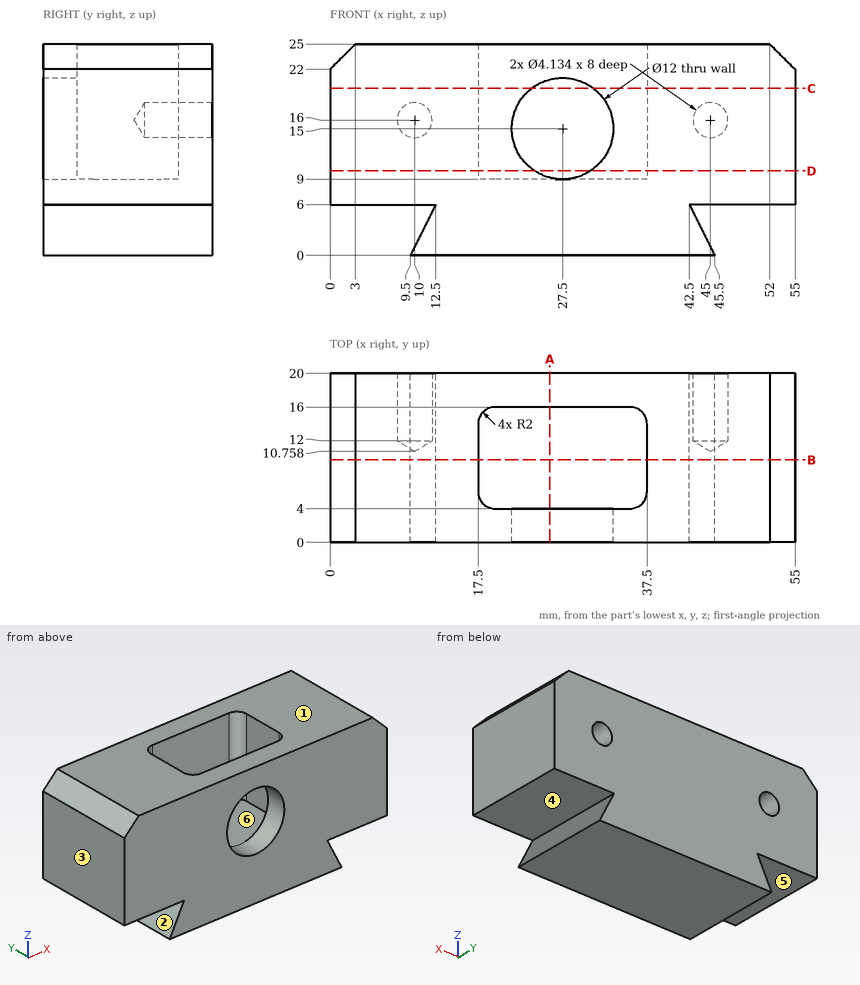
Geometry: see drawing. Coordinates: mm, zero at the bounding-box minimum. A direction names the side the tool comes from. Give positions to 0.01 mm unless a question says otherwise; leave off trailing zeros. Order: outer loops, then holes, each group sorted by start corner. A loop starts at its lowest first (then second) coordinate and runs counter-clockwise, first axis right, second up. Notation, with made-up numbers: (-2, -39) -> (13, -39) arc R14 ccw to (13, -16) -> close; hole circle Ø8 at (-4.5, 28.25). An arc over 180 degrees is marked (long way). Write item = value, one per line.
Q1. Cut plane A-A, the plane x = 26. Output: boundary loops of the cut face in (y, z).
Data:
outline = (0, 0) -> (20, 0) -> (20, 25) -> (16, 25) -> (16, 9) -> (4, 9) -> (4, 9.19) -> (0, 9.19) -> close; (0, 20.81) -> (4, 20.81) -> (4, 25) -> (0, 25) -> close
Q2. Material intervals for line 1 (X direction, y = 14, z = 16); line 2 (X direction, y = 16.25, z = 16); line 3 (Y direction, x = 23, z = 24), sorted ascending. Write a range as from..to.
Data:
line_1 = 0..7.93, 12.07..17.5, 37.5..42.93, 47.07..55
line_2 = 0..7.93, 12.07..42.93, 47.07..55
line_3 = 0..4, 16..20
Q3. Pull-direction query (Z, two-part tool) for the marked faces 1, 2 and 3; classes: released by +Z, released by -Z, zero draft, split by the parting line, or undercut.
Data:
face_1 = released by +Z
face_2 = undercut
face_3 = zero draft
Q4. Pin query (flat end, axial travel): pin 1 (9.5 mm diameter, centred on x = 26, y = 10.5, fed in from +Z); pin 2 (1 mm diameter, centred on y = 7, z = 4.5, fed in from -X). Return the tip coordinate at first contact, or that it passes through.
Data:
pin_1 = 9
pin_2 = 11.5
Q5. Cut plane D-D, the plane z = 10. Output: boundary loops of the cut face in (x, y).
Data:
outline = (0, 0) -> (24.18, 0) -> (24.18, 4) -> (19.5, 4) arc R2 cw to (17.5, 6) -> (17.5, 14) arc R2 cw to (19.5, 16) -> (35.5, 16) arc R2 cw to (37.5, 14) -> (37.5, 6) arc R2 cw to (35.5, 4) -> (30.82, 4) -> (30.82, 0) -> (55, 0) -> (55, 20) -> (0, 20) -> close
Q6. Cut plane B-B, the plane y = 9.75. Output: boundary loops of the cut face in (x, z).
Data:
outline = (0, 6) -> (12.5, 6) -> (9.5, 0) -> (45.5, 0) -> (42.5, 6) -> (55, 6) -> (55, 22) -> (52, 25) -> (37.5, 25) -> (37.5, 9) -> (17.5, 9) -> (17.5, 25) -> (3, 25) -> (0, 22) -> close
Q7. Cut plane C-C, the plane z = 19.75. Output: boundary loops of the cut face in (x, y).
Data:
outline = (0, 0) -> (23.83, 0) -> (23.83, 4) -> (19.5, 4) arc R2 cw to (17.5, 6) -> (17.5, 14) arc R2 cw to (19.5, 16) -> (35.5, 16) arc R2 cw to (37.5, 14) -> (37.5, 6) arc R2 cw to (35.5, 4) -> (31.17, 4) -> (31.17, 0) -> (55, 0) -> (55, 20) -> (0, 20) -> close
Q8. Set-up query: the marked faces 4, 5 and 6. Return all of +Z, -Z, +X, -X, +Y, -Y with unobstructed straight access to the full face (end or side cutting, diameter ignored); none if empty.
Data:
face_4 = +X, +Y, -Y
face_5 = -X, +Y, -Y
face_6 = +Z
